from build123d import *

# Parameters (mm, degrees)
SKETCH_1_W          = 46.8
SKETCH_1_H          = 20
SKETCH_1_R          = 2.55
EXTRUDE_1_DEPTH     = 4.5
CUT_EXTRUDE_1_DEPTH = 8
SKETCH_9_W          = 18
SKETCH_9_H          = 10
EXTRUDE_2_DEPTH     = 10
CUT_EXTRUDE_3_DEPTH = 10
SKETCH_12_R         = 2.75
CUT_EXTRUDE_4_DEPTH = 3


with BuildPart() as part:
    # 草图1 → 凸台-拉伸1 (new body)
    with BuildSketch(Plane.XY):
        with Locations((-1.9, 0)):
            Rectangle(SKETCH_1_W, SKETCH_1_H)
        with Locations((-15.85, 0)):
            Circle(SKETCH_1_R, mode=Mode.SUBTRACT)
        with Locations((15.85, 0)):
            Circle(SKETCH_1_R, mode=Mode.SUBTRACT)
    extrude_1 = extrude(amount=EXTRUDE_1_DEPTH)

    # 草图8 → 切除-拉伸1 (cut)
    with BuildSketch(Plane(origin=(0, 0, 0), x_dir=(-1, 0, 0), z_dir=(0, 0, -1))):
        with BuildLine():
            Line((-8.572541507, 1.430395913), (8.030268199, 1.430395913))
            ThreePointArc((8.030268199, 1.430395913), (9.460664112, 0), (8.030268199, -1.430395913))
            Line((8.030268199, -1.430395913), (-8.572541507, -1.430395913))
            ThreePointArc((-8.572541507, -1.430395913), (-10.00293742, 0), (-8.572541507, 1.430395913))
        make_face()
    cut_extrude_1 = extrude(amount=-CUT_EXTRUDE_1_DEPTH, mode=Mode.SUBTRACT)

    # 镜向1: 凸台-拉伸1 across plane
    add(extrude_1.mirror(Plane.ZX.offset(10)))

    # 镜向3: 切除-拉伸1 across plane
    add(cut_extrude_1.mirror(Plane.ZX.offset(10)), mode=Mode.SUBTRACT)

    # 草图9 → 凸台-拉伸2 (add)
    with BuildSketch(Plane.XY.offset(4.5)):
        with Locations((0, 10)):
            Rectangle(SKETCH_9_W, SKETCH_9_H)
    extrude(amount=EXTRUDE_2_DEPTH)

    # 草图11 → 切除-拉伸3 (cut)
    with BuildSketch(Plane.XZ.offset(-5)):
        with BuildLine():
            Line((-4, 11.5), (4, 11.5))
            ThreePointArc((4, 11.5), (6.5, 9), (4, 6.5))
            Line((4, 6.5), (-4, 6.5))
            ThreePointArc((-4, 6.5), (-6.5, 9), (-4, 11.5))
        make_face()
    extrude(amount=-CUT_EXTRUDE_3_DEPTH, mode=Mode.SUBTRACT)

    # 草图12 → 切除-拉伸4 (cut)
    with BuildSketch(Plane.XY.offset(14.5)):
        with Locations((0, 10)):
            Circle(SKETCH_12_R)
    extrude(amount=-CUT_EXTRUDE_4_DEPTH, mode=Mode.SUBTRACT)


solid = part.part
Check sheet for the modelled part. Datum: model origin and axes. Units: mm. A direction names the side the tool comes from. Round coordinates to 2 decimals unless told otherwise and drop trailing zeros. Write each loop counter-clockwise with the first axis right and the second up, starting at its lowest first coordinate (ties: lowest second). Pieces come first, ordered by that corner, then holes. Notation, with made-up numbers: (-16.5, -21.75) - (40.5, -21.75) arc R22 ccw to (40.5, 12.25) - close; hole circle Ø2 at (86.5, 85). An arc over 180 degrees is marked (long way). Return JSON: item names as keys, results as strings.
Q1. Cross-section at C-C (y = 20). Record the boundary of the cut face in (x, z).
Returned:
{"outline": "(-25.3, 0) - (-18.4, 0) - (-18.4, 4.5) - (-25.3, 4.5) - close; (-13.3, 0) - (-9.46, 0) - (-9.46, 4.5) - (-13.3, 4.5) - close; (10, 0) - (13.3, 0) - (13.3, 4.5) - (10, 4.5) - close; (18.4, 0) - (21.5, 0) - (21.5, 4.5) - (18.4, 4.5) - close"}
Q2. Cross-section at A-A (x = -15.85). Record the boundary of the cut face in (y, z), then the cut area to 3 significant figures.
Returned:
{"outline": "(-10, 0) - (-2.55, 0) - (-2.55, 4.5) - (-10, 4.5) - close; (2.55, 0) - (17.45, 0) - (17.45, 4.5) - (2.55, 4.5) - close; (22.55, 0) - (30, 0) - (30, 4.5) - (22.55, 4.5) - close", "area": "134 mm²"}
Q3. Cross-section at D-D (z = 12.5). Record the boundary of the cut face in (x, y).
Returned:
{"outline": "(-9, 5) - (9, 5) - (9, 15) - (-9, 15) - close; hole circle Ø5.5 at (0, 10)"}
Q4. Access from +Z, -Z, +X, -X, +Y, -Y to the whole of each face (thin tool, end or side, straight path). Record for faces 4 (the flat face through (-1.8, 7.7, 11.5)), 5 (the flat face through (0, -1.43, 2)), 6 (the cylindrical face through (-0.358, 12.727, 13.021)), 7 (the flat face through (0, 5, 12)).
Returned:
{"face 4": "+Y, -Y", "face 5": "+Z, -Z", "face 6": "+Z", "face 7": "+Z, +X, -X, -Y"}
Q5. Depth check by flat-ended pin: P1, Ø8, axis at x = 2, z = 12, coming from the +Y side; P2, Ø4, axis at x = -0.5, y = 9.5, coming from the +Z side; P3, Ø2, axis at y = 12, z = 8, coming from the +X side. Enter the tip coordinate at first touch or a pass-through.
Returned:
{"P1": "stops at y = 15", "P2": "stops at z = 6.5", "P3": "stops at x = 9"}
Q6. Scan lines: L1, parallel to X at y = 20, z = 3.4; L2, parallel to Y at x = 15.85, z = 1.4; L3, parallel to Y at x = 5.5, z = 4.25. Record each from-to range of solid material in increasing order. Write a range as from..to.
Returned:
{"L1": "x = -25.3..-18.4, -13.3..-9.46, 10..13.3, 18.4..21.5", "L2": "y = -10..-2.55, 2.55..17.45, 22.55..30", "L3": "y = -10..-1.43, 1.43..18.57, 21.43..30"}
Q7. Draft check along Z on faces 1 (the flat face through (-13, 10, 4.5)), 2 (the cylindrical face through (-13.42, 19.23, 2.22)), 3 (the flat face through (0, 10, 6.5)). Enter one of: released by +Z, released by -Z, zero draft, split by the parting line, or undercut.
Returned:
{"face 1": "released by +Z", "face 2": "zero draft", "face 3": "undercut"}
Q8. Cross-section at B-B (z = 7.5). Record the boundary of the cut face in (x, y).
Returned:
{"outline": "(-9, 5) - (-6, 5) - (-6, 15) - (-9, 15) - close; (6, 5) - (9, 5) - (9, 15) - (6, 15) - close"}
